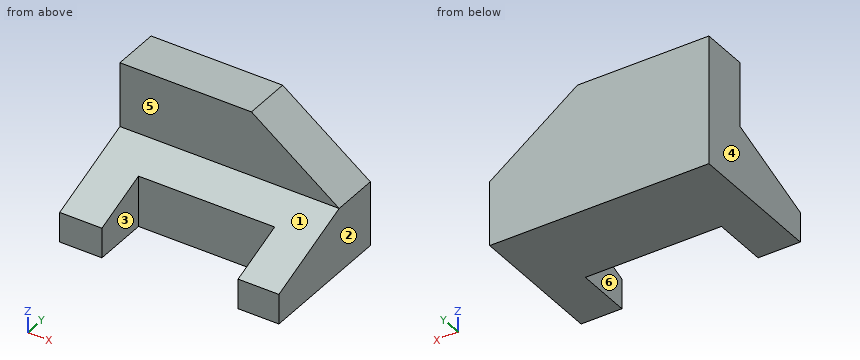
```python
from build123d import *

# Parameters (mm, degrees)
F0_W     = 20.443046
F0_H     = 28
F1_DEPTH = 95
F3_DEPTH = 25
F4_W     = 59
F4_H     = 24
F5_DEPTH = 25


with BuildPart() as f1:
    # F0 (on Right) → F1 (new body)
    with BuildSketch(Plane.YZ):
        with Locations((-4.743823, 8.828466)):
            Rectangle(F0_W, F0_H)
        Polygon((-54.5223, -20.171534), (-54.5223, -33.171534), (5.4777, -33.171534), (5.4777, -5.171534), (-14.965346, -5.171534), align=None)
    extrude(amount=-F1_DEPTH)

    # F2 (on face) → F3 (cut)
    with BuildSketch(Plane.XZ.offset(14.965346)):
        Polygon((0, 22.828466), (-38, 22.828466), (0, -5.171534), align=None)
    extrude(amount=-F3_DEPTH, mode=Mode.SUBTRACT)

    # F4 (on face) → F5 (cut)
    with BuildSketch(Plane(origin=(0, 0, -33.171534), x_dir=(1, 0, 0), z_dir=(0, 0, -1))):
        with Locations((-47.190733, 42.5223)):
            Rectangle(F4_W, F4_H)
    extrude(amount=-F5_DEPTH, mode=Mode.SUBTRACT)


solid = f1.part
```
Geometry: final body of the model. Coordinates: model frame, mm. Face numbers are marked on the shaded views. A direction names the side the tool comes from. Round coordinates to 2 decimals unless told otherwise and drop trailing zeros. Loops run counter-clockwise (first coordinate to the right, second up) from the corner with the lowest first, then second, coordinate; pieces in that order, holes last. Notation, with made-up numbers: (31, -2) -> (80, -2) arc R15 ccw to (80, 6) -> close; hole circle Ø4 at (-22, 75). An arc over 180 degrees is marked (long way). Use one line per item in the form item = value.
Item 1: Access query for the marked faces 4, 5 and 6. Directions: +Z, -Z, +X, -X, +Y, -Y. A direction counts if a zero-diameter tool reaches every point of the face in a straight line with its end or side. Return the directions, or none.
Evaluation:
face_4 = +Z, -Z, -X, +Y, -Y
face_5 = +Z, +X, -X, -Y
face_6 = +Z, -Z, -Y
Item 2: Material intervals for probe 1 along X at (y, z) = (-47.5, -24); probe 2 along Y at (x, z) = (-42, -17); probe 3 along Y at (x, z) = (-47.5, 13), sorted ascending.
Evaluation:
probe_1 = -95 to -76.69, -17.69 to 0
probe_2 = -30.52 to 5.48
probe_3 = -14.97 to 5.48
Item 3: Cut plane A-A on z = -29. Output: boundary loops of the cut face in (x, y), then the cut area to 3 significant figures.
Evaluation:
outline = (-95, -54.52) -> (-76.69, -54.52) -> (-76.69, -30.52) -> (-17.69, -30.52) -> (-17.69, -54.52) -> (0, -54.52) -> (0, 5.48) -> (-95, 5.48) -> close
area = 4,280 mm2
Item 4: Cut plane C-C on x = -79.5. Output: boundary loops of the cut face in (y, z).
Evaluation:
outline = (-54.52, -33.17) -> (5.48, -33.17) -> (5.48, 22.83) -> (-14.97, 22.83) -> (-14.97, -5.17) -> (-54.52, -20.17) -> close
Item 5: Contact query for flat-ended pins moving along their axis: pin 1 Ø10 at (x, z) = (-25, 13.5) entering from -Y; pin 2 Ø6.5 at (x, z) = (-48.5, -24) entering from -Y; pin 3 Ø2 at (x, y) = (-30.5, -29) entering from +Z. Output: stop coordinate, or through.
Evaluation:
pin_1 = -14.97
pin_2 = -30.52
pin_3 = -10.11
Item 6: Cut plane B-B on y = -44. Output: boundary loops of the cut face in (x, z).
Evaluation:
outline = (-95, -33.17) -> (-76.69, -33.17) -> (-76.69, -16.18) -> (-95, -16.18) -> close; (-17.69, -33.17) -> (0, -33.17) -> (0, -16.18) -> (-17.69, -16.18) -> close
Item 7: Draft query along X for the marked faces 1, 2 and 3. Return one class per face: released by +X, released by -X, zero draft, split by the parting line, or undercut.
Evaluation:
face_1 = zero draft
face_2 = released by +X
face_3 = undercut
Item 8: Cut plane D-D on y = -6.5. Output: boundary loops of the cut face in (x, z).
Evaluation:
outline = (-95, -33.17) -> (0, -33.17) -> (0, -5.17) -> (-38, 22.83) -> (-95, 22.83) -> close
